Check sheet for the modelled part. Datum: model origin and axes. Units: mm. Face numbers are marked on the shaded views. A direction names the side the tool comes from. Round coordinates to 2 decimals unless told otherwise and drop trailing zeros. Write each loop counter-clockwise with the first axis right and the second up, starting at its lowest first coordinate (ties: lowest second). Pieces come first, ordered by that corner, then holes.
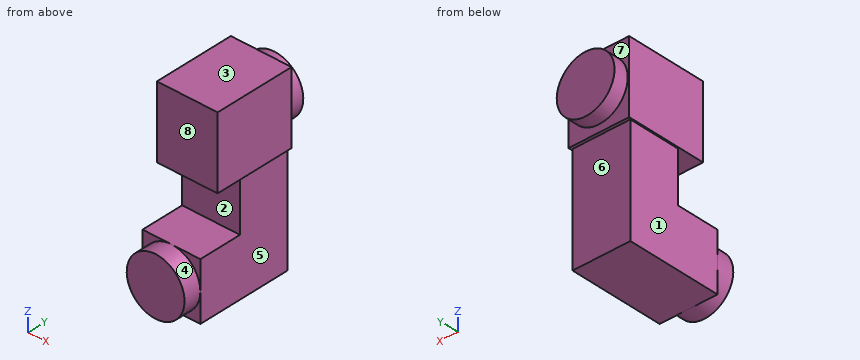
from build123d import *

# Parameters (mm, degrees)
ESQUISSE1_W        = 25
ESQUISSE1_H        = 28
BOSS_EXTRU_1_DEPTH = 21
ESQUISSE2_W        = 20
ESQUISSE2_H        = 18
BOSS_EXTRU_2_DEPTH = 37.5
ESQUISSE3_W        = 20
ESQUISSE3_H        = 20
BOSS_EXTRU_3_DEPTH = 15
ESQUISSE5_R        = 10
BOSS_EXTRU_4_DEPTH = 5
ESQUISSE6_R        = 10
BOSS_EXTRU_5_DEPTH = 6


with BuildPart() as part:
    # Esquisse1 → Boss.-Extru.1 (new body)
    with BuildSketch(Plane(origin=(0, 0, 0), x_dir=(0, 0, -1), z_dir=(1, 0, 0))):
        with Locations((156.893217971, 169.300046999)):
            Rectangle(ESQUISSE1_W, ESQUISSE1_H)
    extrude(amount=BOSS_EXTRU_1_DEPTH)

    # Esquisse2 → Boss.-Extru.2 (add)
    with BuildSketch(Plane(origin=(0, 0, -169.393217971), x_dir=(-1, 0, 0), z_dir=(0, 0, -1))):
        with Locations((-10.5, 173.300046999)):
            Rectangle(ESQUISSE2_W, ESQUISSE2_H)
    extrude(amount=BOSS_EXTRU_2_DEPTH)

    # Esquisse3 → Boss.-Extru.3 (add)
    with BuildSketch(Plane.XZ.offset(-164.300046999)):
        with Locations((10.5, -196.893217971)):
            Rectangle(ESQUISSE3_W, ESQUISSE3_H)
    extrude(amount=BOSS_EXTRU_3_DEPTH)

    # Esquisse5 → Boss.-Extru.4 (add)
    with BuildSketch(Plane(origin=(0, 183.300046999, 0), x_dir=(1, 0, 0), z_dir=(0, 1, 0))):
        with Locations(Location((10.5, 156.893217971, 0), (0, 0, 270))):
            Circle(ESQUISSE5_R)
    extrude(amount=BOSS_EXTRU_4_DEPTH)

    # Esquisse6 → Boss.-Extru.5 (add)
    with BuildSketch(Plane(origin=(0, 149.300046999, 0), x_dir=(-1, 0, 0), z_dir=(0, -1, 0))):
        with Locations(Location((-10.5, 196.893217971, 0), (0, 0, 90))):
            Circle(ESQUISSE6_R)
    extrude(amount=BOSS_EXTRU_5_DEPTH)


solid = part.part
1. Sectioned sample at D-D, the plane y = 153.5. Enter the section's corners in (x, z).
2. Sectioned sample at C-C, the plane x = 4.25. Enter the section's corners in (y, z), plus the area to 3 significant figures.
3. Sectioned sample at A-A, the plane y = 179. Enter the section's corners in (x, z), plus the area to 4 significant figures.
4. Scan lines: line 1 along Z through (x, y) = (8.5, 162.5); line 2 along X through (y, z) = (168.5, -181); line 3 along Y through (x, z) = (15.5, -170). Record each from-to range of solid material in increasing order.
5. Go/stop test with flat-tipped pins: pin 1 (3 mm diameter, centred on x = 2.5, z = -174.5, fed in from -Y); pin 2 (16.5 mm diameter, centred on y = 167.5, z = -193.5, fed in from +X); pin 3 (12 mm diameter, centred on y = 172.5, z = -184.5, fed in from -X). Record where each tip stops, or that it passes through.
6. Release check for a two-part mould opening along Z. For the marked faces 1, 2 and 3 record: released by +Z, released by -Z, zero draft, split by the parting line, or undercut.
7. Set-up check for the marked faces 4, 5, 6, 7 and 8: record each of +Z, -Z, +X, -X, +Y, -Y from which the full face is reachable in a straight line by a thin tool's end or side.
8. Sectioned sample at B-B, the plane z = -162.5. Enter the section's corners in (x, y), plus the area to 3 significant figures.
Computed values:
1. outline: (0.5, -206.89) - (20.5, -206.89) - (20.5, -186.89) - (0.5, -186.89) - close
2. outline: (143.3, -204.7) - (149.3, -204.7) - (149.3, -206.89) - (182.3, -206.89) - (182.3, -169.39) - (183.3, -169.39) - (183.3, -164.7) - (188.3, -164.7) - (188.3, -149.09) - (183.3, -149.09) - (183.3, -144.39) - (155.3, -144.39) - (155.3, -169.39) - (164.3, -169.39) - (164.3, -186.89) - (149.3, -186.89) - (149.3, -189.09) - (143.3, -189.09) - close
2. area: 1,850 mm2
3. outline: (0, -169.39) - (0.5, -169.39) - (0.5, -206.89) - (20.5, -206.89) - (20.5, -169.39) - (21, -169.39) - (21, -144.39) - (0, -144.39) - close
3. area: 1,275 mm2
4. line 1: z = -206.89 to -186.89, -169.39 to -144.39
4. line 2: x = 0.5 to 20.5
4. line 3: y = 164.3 to 182.3
5. pin 1: stops at y = 164.3
5. pin 2: stops at x = 20.5
5. pin 3: stops at x = 0.5
6. face 1: zero draft
6. face 2: undercut
6. face 3: released by +Z
7. face 4: -Y
7. face 5: -Z, +X, +Y, -Y
7. face 6: -Z, +X, -X, +Y
7. face 7: +Y
7. face 8: +Z, +X, -X, -Y
8. outline: (0, 155.3) - (21, 155.3) - (21, 183.3) - (18.78, 183.3) - (18.78, 188.3) - (2.22, 188.3) - (2.22, 183.3) - (0, 183.3) - close
8. area: 671 mm2
